Design review of the part built by this model. Coordinates are the model's own, in mm. Coordinates: 2 decimals unless noted, no trailing zeros. Loops run counter-clockwise (first coordinate to the right, second up) from the corner with the lowest first, then second, coordinate; pieces in that order, holes last. Notation, with made-up numbers: (48.25, 50.5) -> (67.25, 50.5) arc R34 cw to (67.25, 81.5) -> close; hole circle Ø9 at (34.5, -2.75). An arc over 180 degrees is marked (long way). Answer as a JSON object with one key per item and string values.
```python
from build123d import *

# Parameters (mm, degrees)
SKETCH1_W                  = 55
SKETCH1_H                  = 55
BOSS_EXTRUDE1_DEPTH        = 2.5
F_4_8_4_8_DIAMETER_HOLE1_D = 4.8
LPATTERN1_COUNT            = 2
LPATTERN1_PITCH            = 36
LPATTERN1_COUNT_DIR2       = 2
LPATTERN1_PITCH_DIR2       = 36
SKETCH4_R                  = 2
CUT_EXTRUDE1_DEPTH         = 40.210967853


with BuildPart() as part:
    # Sketch1 → Boss-Extrude1 (new, symmetric)
    with BuildSketch(Plane.XY):
        Rectangle(SKETCH1_W, SKETCH1_H)
    extrude(amount=BOSS_EXTRUDE1_DEPTH, both=True)

    # Ø4.8 (4.8) Diameter Hole1 (through all)
    with Locations(Plane.XY.offset(2.5)):
        with Locations((18, 18)):
            f_4_8_4_8_diameter_hole1 = Hole(F_4_8_4_8_DIAMETER_HOLE1_D / 2)

    # LPattern1: 4.8 _4.8_ Diameter Hole1 2 × 2
    with Locations(*[(-i * LPATTERN1_PITCH, -j * LPATTERN1_PITCH_DIR2, 0) for i in range(LPATTERN1_COUNT) for j in range(LPATTERN1_COUNT_DIR2) if (i, j) != (0, 0)]):
        add(f_4_8_4_8_diameter_hole1, mode=Mode.SUBTRACT)

    # Sketch4 → Cut-Extrude1 (cut, through all)
    with BuildSketch(Plane.XY.offset(2.5)):
        with Locations((0, 15)):
            Circle(SKETCH4_R)
        with Locations((0, -15)):
            Circle(SKETCH4_R)
    extrude(amount=-CUT_EXTRUDE1_DEPTH, mode=Mode.SUBTRACT)


solid = part.part
```
1) Add section A-A, the plane y = -18. Give the boundary of the cut face in (x, z).
Completed:
{"outline": "(-27.5, -2.5) -> (-20.4, -2.5) -> (-20.4, 2.5) -> (-27.5, 2.5) -> close; (-15.6, -2.5) -> (15.6, -2.5) -> (15.6, 2.5) -> (-15.6, 2.5) -> close; (20.4, -2.5) -> (27.5, -2.5) -> (27.5, 2.5) -> (20.4, 2.5) -> close"}
2) Add section C-C, the plane z = 0.75. Give the boundary of the cut face in (x, y), and give its area (3 significant figures).
Completed:
{"outline": "(-27.5, -27.5) -> (27.5, -27.5) -> (27.5, 27.5) -> (-27.5, 27.5) -> close; hole circle Ø4.8 at (-18, -18); hole circle Ø4.8 at (-18, 18); hole circle Ø4 at (0, -15); hole circle Ø4 at (0, 15); hole circle Ø4.8 at (18, -18); hole circle Ø4.8 at (18, 18)", "area": "2,930 mm²"}
3) The part is to be moulded in two halves that separate along Y. For faces 1 (the flat face through (0, 27.5, 0)), 2 (the flat face through (0, -27.5, 0)), 3 (the cylindrical face through (0, 17, 0)), 4 (the cylindrical face through (-15.602, -17.894, -0.035)), say which applies: pulls with the +Y half, pulls with the -Y half, needs draft (parallel to the pull), parting line crosses it, or undercut.
Completed:
{"face 1": "pulls with the +Y half", "face 2": "pulls with the -Y half", "face 3": "undercut", "face 4": "undercut"}
4) Add section B-B, the plane x = 0. Give the boundary of the cut face in (y, z), and give its area (3 significant figures).
Completed:
{"outline": "(-27.5, -2.5) -> (-17, -2.5) -> (-17, 2.5) -> (-27.5, 2.5) -> close; (-13, -2.5) -> (13, -2.5) -> (13, 2.5) -> (-13, 2.5) -> close; (17, -2.5) -> (27.5, -2.5) -> (27.5, 2.5) -> (17, 2.5) -> close", "area": "235 mm²"}
5) Wall thickness on probe 1 along Y at (x, z) = (0, -2.1); probe 2 along Y at (x, z) = (18, 1.2); probe 3 along X at (y, z) = (19.5, 0.8): over which ranges is each line inside the solid? List them lowest first.
Completed:
{"probe 1": "-27.5 to -17, -13 to 13, 17 to 27.5", "probe 2": "-27.5 to -20.4, -15.6 to 15.6, 20.4 to 27.5", "probe 3": "-27.5 to -19.87, -16.13 to 16.13, 19.87 to 27.5"}
